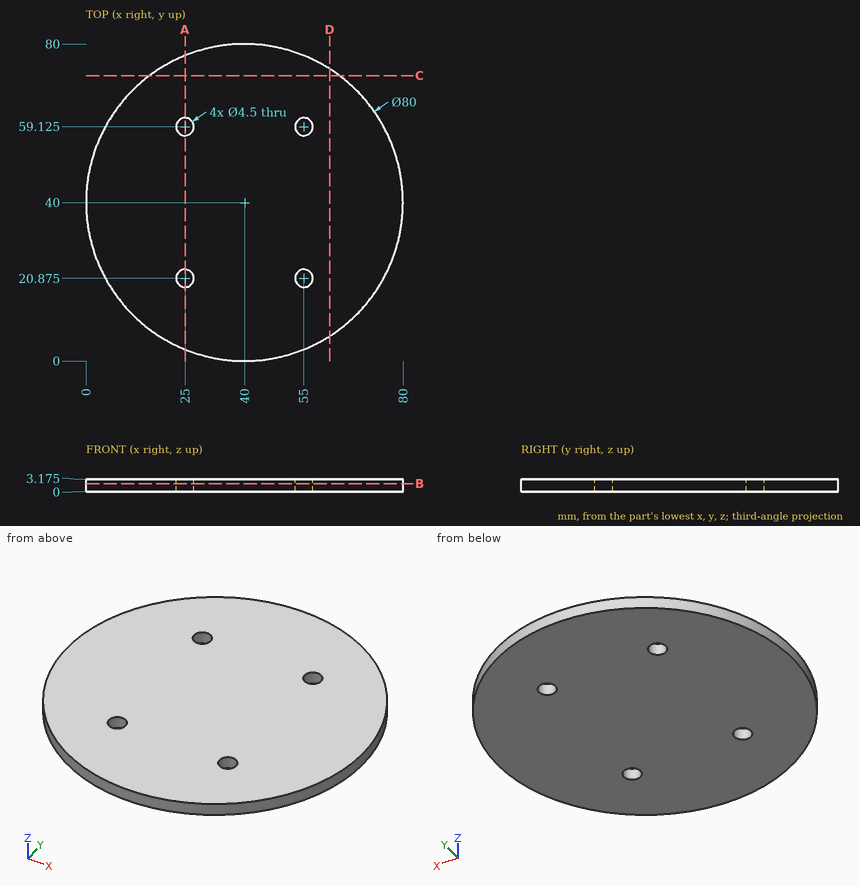
Design review of the part shown in the three views and the two pictorial views. Dimensions are in mm from the part's minimum x, y and z. Round coordinates to 2 decimals unless told otherwise and drop trailing zeros. Order: outer loops, then holes, each group sorted by start corner. A loop starts at its lowest first (then second) coordinate and runs counter-clockwise, first axis right, second up.
(1) Take a section at B-B, the plane z = 2. State the section outline as (x, y) points (3 decimals).
Working result:
outline: circle Ø80 at (40, 40); hole circle Ø4.5 at (25, 20.875); hole circle Ø4.5 at (25, 59.125); hole circle Ø4.5 at (55, 20.875); hole circle Ø4.5 at (55, 59.125)
(2) For P1, Ø2.5, axis at x = 25, y = 59.125, coming from the +Z side, flat-tipped, find the tip position at first contact; note if it passes through.
Working result:
P1: passes through
(3) Take a section at A-A, the plane x = 25. State the section outline as (y, z) points (3 decimals).
Working result:
outline: (2.919, 0) - (18.625, 0) - (18.625, 3.175) - (2.919, 3.175) - close; (23.125, 0) - (56.875, 0) - (56.875, 3.175) - (23.125, 3.175) - close; (61.375, 0) - (77.081, 0) - (77.081, 3.175) - (61.375, 3.175) - close
(4) Take a section at D-D, the plane x = 61.5. State the section outline as (y, z) points (3 decimals).
Working result:
outline: (6.269, 0) - (73.731, 0) - (73.731, 3.175) - (6.269, 3.175) - close
(5) Wall thickness on L1, parallel to Y at x = 25, z = 1.75 (3 decimals); L2, parallel to X at y = 21, z = 2.35; L3, parallel to Y at x = 56.5, z = 2.55: over which ranges is each line inside the solid? List them lowest first.
Working result:
L1: y = 2.919 to 18.625, 23.125 to 56.875, 61.375 to 77.081
L2: x = 4.8 to 22.75, 27.25 to 52.75, 57.25 to 75.2
L3: y = 3.56 to 19.2, 22.55 to 57.45, 60.8 to 76.44
(6) Take a section at C-C, the plane y = 72. State the section outline as (x, z) points (3 decimals), plus the area to 3 significant figures.
Working result:
outline: (16, 0) - (64, 0) - (64, 3.175) - (16, 3.175) - close
area: 152 mm2
